from build123d import *

# Parameters (mm, degrees)
SKETCH_1_R          = 1.75
EXTRUDE_1_DEPTH     = 10
SKETCH_2_R          = 1.75
CUT_EXTRUDE_1_DEPTH = 21


with BuildPart() as part:
    # 草图1 → 凸台-拉伸1 (new body)
    with BuildSketch(Plane(origin=(0, 0, 0), x_dir=(1, 0, 0), z_dir=(0, 1, 0))):
        with BuildLine():
            Line((-102.099280991, 5.948332783), (-79.599280991, 5.948332783))
            ThreePointArc((-79.599280991, 5.948332783), (-73.099280991, -0.551667217), (-79.599280991, -7.051667217))
            Line((-79.599280991, -7.051667217), (-102.099280991, -7.051667217))
            ThreePointArc((-102.099280991, -7.051667217), (-108.599280991, -0.551667217), (-102.099280991, 5.948332783))
        make_face()
        with Locations(Location((-105.419280991, -0.551667217, 0), (0, 0, 270))):
            Circle(SKETCH_1_R, mode=Mode.SUBTRACT)
        with Locations(Location((-76.279280991, -0.551667217, 0), (0, 0, 270))):
            Circle(SKETCH_1_R, mode=Mode.SUBTRACT)
    extrude(amount=EXTRUDE_1_DEPTH)

    # 草图2 → 切除-拉伸1 (cut)
    with BuildSketch(Plane(origin=(0, 0, -5.948332783), x_dir=(-1, 0, 0), z_dir=(0, 0, -1))):
        with Locations((99.099280991, 5)):
            Circle(SKETCH_2_R)
        with Locations((82.599280991, 5)):
            Circle(SKETCH_2_R)
    extrude(amount=-CUT_EXTRUDE_1_DEPTH, mode=Mode.SUBTRACT)


solid = part.part
Work out the finished part from the listing and answer in its coordinate system (mm). Give positions to 0.01 mm unless a question says otherwise; leave off trailing zeros. Write each loop counter-clockwise with the first axis right and the second up, starting at its lowest first coordinate (ties: lowest second). Pieces come first, ordered by that corner, then holes. Notation, with made-up numbers: M -36.75,23.25 L 14.25,23.25 A14 cw 14.25,29.25 Z; hole C 9.5,20 d1. An arc over 180 degrees is marked long. Answer as CSV lines item,"result".
Q1. Given P1, Ø4, axis at y = 6, z = 3, coming from the +X side; P2, Ø1.5, axis at x = -103.5, y = 1, coming from the -Z side; P3, Ø4, axis at y = 5.5, z = -4, coming from the -X side, each flat-ended and moving along its own axis, determine where each tip first touches the part or whether it passes through.
A:
P1,"stops at x = -73.11"
P2,"stops at z = -5.92"
P3,"stops at x = -108.08"
Q2. A cutting plane is placed at D-D on y = 2. Write down the section's boundary in (x, z), plus the area to 3 significant figures.
A:
outline,"M -102.1,-5.95 L -79.6,-5.95 A6.5 ccw -79.6,7.05 L -102.1,7.05 A6.5 ccw Z; hole C -105.42,0.55 d3.5; hole C -76.28,0.55 d3.5"
area,"406 mm²"
Q3. A cutting plane is placed at B-B on z = 0. Write down the section's boundary in (x, y), plus the area to 3 significant figures.
A:
outline,"M -108.58,0 L -107.08,0 L -107.08,10 L -108.58,10 Z; M -103.76,0 L -77.94,0 L -77.94,10 L -103.76,10 Z; M -74.62,0 L -73.12,0 L -73.12,10 L -74.62,10 Z; hole C -99.1,5 d3.5; hole C -82.6,5 d3.5"
area,"269 mm²"
Q4. Find the intervals of material crossed by probe 1 along Y at (x, z) = (-99, -4); probe 2 along X at (y, z) = (4.75, 2.5); probe 3 along X at (y, z) = (1.5, 2), in increasing order. Write a range as [from, to].
A:
probe 1,"y = [0, 3.25], [6.75, 10]"
probe 2,"x = [-108.3, -100.83], [-97.37, -84.33], [-80.87, -73.4]"
probe 3,"x = [-108.44, -106.4], [-104.44, -77.26], [-75.3, -73.26]"
Q5. The mould has two halves that part along Y. Classify faces 1 (the flat face through (-91, 5, -5.948)), 2 (the cylindrical face through (-80.85, 5.08, 0.46)), 3 (the flat face through (-91, 10, 0)), 4 (the cylindrical face through (-98.72, 3.29, 0.46)): +Y half, -Y half, draft (parallel to the pull), parting line (faces both ways), or undercut.
A:
face 1,"draft"
face 2,"undercut"
face 3,"+Y half"
face 4,"undercut"
Q6. A cutting plane is placed at A-A on y = 5. Write down the section's boundary in (x, z), plus the area to 3 significant figures.
A:
outline,"M -102.1,-5.95 L -100.85,-5.95 L -100.85,7.05 L -102.1,7.05 A6.5 ccw Z; M -97.35,-5.95 L -84.35,-5.95 L -84.35,7.05 L -97.35,7.05 Z; M -80.85,-5.95 L -79.6,-5.95 A6.5 ccw -79.6,7.05 L -80.85,7.05 Z; hole C -105.42,0.55 d3.5; hole C -76.28,0.55 d3.5"
area,"315 mm²"
Q7. A cutting plane is placed at C-C on z = 3. Write down the section's boundary in (x, y).
A:
outline,"M -108.12,0 L -73.58,0 L -73.58,10 L -108.12,10 Z; hole C -99.1,5 d3.5; hole C -82.6,5 d3.5"
